from build123d import *

# Parameters (mm, degrees)
SKETCH1_W                = 160
SKETCH1_H                = 60
BOSS_EXTRUDE1_DEPTH      = 5
BOSS_EXTRUDE3_DEPTH      = 14.3
BOSS_EXTRUDE3_DEPTH_BACK = 14.3
SKETCH8_W                = 20
SKETCH8_H                = 23
CUT_EXTRUDE1_REACH       = 134.986
BOSS_EXTRUDE4_DEPTH      = 60
CUT_EXTRUDE2_START       = -71.5
SKETCH11_W               = 45
SKETCH11_H               = 40
CUT_EXTRUDE2_DEPTH       = 71.5
SKETCH12_W               = 24.082620142
SKETCH12_H               = 45
CUT_EXTRUDE3_DEPTH       = 24
SKETCH13_R               = 3.5
SKETCH13_R_2             = 1.7
CUT_EXTRUDE4_DEPTH       = 7.417379858
SKETCH14_R               = 3.5
BOSS_EXTRUDE5_DEPTH      = 60
SKETCH16_W               = 47
SKETCH16_H               = 47.898935067
CUT_EXTRUDE6_DEPTH       = 107.5
CUT_EXTRUDE7_DEPTH       = 28.5
CUT_EXTRUDE7_DEPTH_BACK  = 28.5
SKETCH17_R               = 7


with BuildPart() as part:
    # Sketch1 → Boss-Extrude1 (new body)
    with BuildSketch(Plane(origin=(0, 0, 0), x_dir=(1, 0, 0), z_dir=(0, 1, 0))):
        Rectangle(SKETCH1_W, SKETCH1_H)
    extrude(amount=BOSS_EXTRUDE1_DEPTH)

    # Sketch8 → Boss-Extrude3 (add, two sides: drawn at the far end of the back side and taken through both)
    with BuildSketch(Plane.XY.offset(-BOSS_EXTRUDE3_DEPTH_BACK)):
        with Locations((-37.5, -11.5)):
            Rectangle(SKETCH8_W, SKETCH8_H)
        with BuildLine():
            Line((-45, -18.5), (-30, -18.5))
            ThreePointArc((-30, -18.5), (-28.5, -20), (-30, -21.5))
            Line((-30, -21.5), (-45, -21.5))
            ThreePointArc((-45, -21.5), (-46.5, -20), (-45, -18.5))
        make_face(mode=Mode.SUBTRACT)
        with BuildLine():
            Line((-45, -0.9), (-30, -0.9))
            ThreePointArc((-30, -0.9), (-28.5, -2.4), (-30, -3.9))
            Line((-30, -3.9), (-45, -3.9))
            ThreePointArc((-45, -3.9), (-46.5, -2.4), (-45, -0.9))
        make_face(mode=Mode.SUBTRACT)
    extrude(amount=BOSS_EXTRUDE3_DEPTH + BOSS_EXTRUDE3_DEPTH_BACK)

    # Cut-Extrude1: up to this face of the body (flat: up to its plane)
    cut_extrude1_end = Plane(part.part.faces().sort_by_distance((-27.5, -11.5, 0))[0])
    # Sketch9 → Cut-Extrude1 (cut, up to the picked face)
    with BuildSketch(Plane.ZY.offset(47.5), mode=Mode.PRIVATE) as cut_extrude1_sk1:
        Polygon((-9.3, -23), (9.3, -23), (9.3, 0), (-9.3, 0), (-9.3, -9.4), (-11.3, -9.4), (-11.3, -13.4), (-9.3, -13.4), align=None)
    cut_extrude1_tool1 = split(extrude(cut_extrude1_sk1.sketch, amount=-CUT_EXTRUDE1_REACH, mode=Mode.PRIVATE), bisect_by=cut_extrude1_end, keep=Keep.BOTH, mode=Mode.PRIVATE)
    add(cut_extrude1_tool1.solids().sort_by(Axis((-47.5, -11.498164, -0.189078), (1, 0, 0)))[0], mode=Mode.SUBTRACT)

    # Sketch10 → Boss-Extrude4 (add)
    with BuildSketch(Plane.XY.offset(30)):
        Polygon((-72.5, 69), (-8.5, 5), (-19.106601718, 5), (-70, 55.893398282), (-70, 5), (-72.5, 5), (-80, 5), (-80, 69), align=None)
    extrude(amount=-BOSS_EXTRUDE4_DEPTH)

    # Sketch11 → Cut-Extrude2 (cut)
    with BuildSketch(Plane.ZY.offset(80).offset(CUT_EXTRUDE2_START)):
        with Locations((0, 25)):
            Rectangle(SKETCH11_W, SKETCH11_H)
    extrude(amount=CUT_EXTRUDE2_DEPTH, mode=Mode.SUBTRACT)

    # Sketch12 → Cut-Extrude3 (cut)
    with BuildSketch(Plane(origin=(0, 69, 0), x_dir=(1, 0, 0), z_dir=(0, 1, 0))):
        with Locations((-60.541310071, 0)):
            Rectangle(SKETCH12_W, SKETCH12_H)
    extrude(amount=-CUT_EXTRUDE3_DEPTH, mode=Mode.SUBTRACT)

    # Sketch13 → Cut-Extrude4 (cut)
    with BuildSketch(Plane.ZY.offset(80)):
        with Locations((0, 57)):
            Circle(SKETCH13_R)
        with Locations((-8.5, 57)):
            Circle(SKETCH13_R_2)
        with Locations((8.5, 57)):
            Circle(SKETCH13_R_2)
    extrude(amount=-CUT_EXTRUDE4_DEPTH, mode=Mode.SUBTRACT)

    # Sketch14 → Boss-Extrude5 (add)
    with BuildSketch(Plane.XY.offset(30)):
        with BuildLine():
            Line((80, 0), (66.844135363, -38.995809861))
            ThreePointArc((66.844135363, -38.995809861), (55, -47.500001557), (43.155864637, -38.995809861))
            Line((43.155864637, -38.995809861), (30, 0))
            Line((30, 0), (37.5, 0))
            Line((37.5, 0), (46.28476615, -26.03926689))
            ThreePointArc((46.28476615, -26.03926689), (55, -22.499998443), (63.71523385, -26.03926689))
            Line((63.71523385, -26.03926689), (72.5, 0))
            Line((72.5, 0), (80, 0))
        make_face()
        with Locations((55, -35)):
            Circle(SKETCH14_R, mode=Mode.SUBTRACT)
    extrude(amount=-BOSS_EXTRUDE5_DEPTH)

    # Sketch16 → Cut-Extrude6 (cut)
    with BuildSketch(Plane(origin=(80, 0, 0), x_dir=(0, 0, -1), z_dir=(1, 0, 0))):
        with Locations((0, -23.949467534)):
            Rectangle(SKETCH16_W, SKETCH16_H)
    extrude(amount=-CUT_EXTRUDE6_DEPTH, mode=Mode.SUBTRACT)

    # Sketch17 → Cut-Extrude7 (cut, two sides: drawn at the far end of the back side and taken through both)
    with BuildSketch(Plane.XY.offset(-CUT_EXTRUDE7_DEPTH_BACK)):
        with Locations((55, -35)):
            Circle(SKETCH17_R)
    extrude(amount=CUT_EXTRUDE7_DEPTH + CUT_EXTRUDE7_DEPTH_BACK, mode=Mode.SUBTRACT)


solid = part.part
The listing builds one solid part. Answer for the finished solid, in the listing's coordinates (mm). A direction names the side the tool comes from. Round coordinates to 2 decimals unless told otherwise and drop trailing zeros. Write each loop counter-clockwise with the first axis right and the second up, starting at its lowest first coordinate (ties: lowest second). Pieces come first, ordered by that corner, then holes. Notation, with made-up numbers: M 71,84.25 L 110,84.25 A33 ccw 110,114.25 Z; hole C -23.75,-3.5 d11. An arc over 180 degrees is marked long. Write each question's results on one line, items separated by ' | '. Start each with the question number.
Item 1: For faces 1 (the face through (58, -38, 28.5)), 2 (the face through (-27.5, -12, 12)), 3 (the face through (68.046, -13.202, -26.705)), 4 (the face through (55, -24, -23.5)), 5 (the face through (-76, 45, 0)), determine the directions among +Z, -Z, +X, -X, +Y, -Y from which every point of the face is accessible in a straight line to the end or side of a thin tool.
Item 2: A cutting plane is placed at C-C on x = 53.5. Write down the section's boundary in (y, z).
Item 3: A cutting plane is placed at D-D on x = -58. Write down the section's boundary in (y, z), and give its area (3 significant figures).
Item 4: A cutting plane is placed at B-B on x = -11. Write down the section's boundary in (y, z), and give its area (4 significant figures).
Item 5: Flat-ended cylindrical pins translate along their axes: pin 1 Ø6 at (x, z) = (53.5, -16.5) entering from +Y; pin 2 Ø4 at (y, z) = (19.5, 27) entering from +X; pin 3 Ø5.5 at (x, z) = (-36.5, -11.5) entering from -Y. Find the tip coordinate at first contact, or state that the pin passes through.
Item 6: For a pull along Z with two mould halves and no side action, classify faces 6 (the face through (-38, -12, 9.3)), 7 (the face through (52.42, -32.635, -29.24)), 8 (the face through (-38, -11, -14.3)), 9 (the face through (-72.583, 57, 5)) as pulls with the +Z half, pulls with the -Z half, needs draft (parallel to the pull), parting line crosses it, or undercut.
Item 7: A cutting plane is placed at A-A on y = -35. Write down the section's boundary in (x, z), and give its area (3 significant figures).
Item 8: Straight lines are drawn through the part: L1, parallel to Y at x = 55, z = -24.6; L2, parallel to Y at x = -78.5, z = -8.5; L3, parallel to Y at x = 59, z = 21. For each, find the intervals that lie inside material, in ascending order. Write a range as [from, to].
Check sheet entries:
1) face 1: none | face 2: +Z, -Z, +X, -Y | face 3: +Z, -Z | face 4: +X, -X, -Y | face 5: +X, -X
2) outline: M -47.41,-30 L -38.16,-30 L -38.16,-28.5 L -41.84,-28.5 L -41.84,-23.5 L -47.41,-23.5 Z; M -47.41,23.5 L -41.84,23.5 L -41.84,28.5 L -38.16,28.5 L -38.16,30 L -47.41,30 Z; M -31.84,-30 L -22.59,-30 L -22.59,-23.5 L -28.16,-23.5 L -28.16,-28.5 L -31.84,-28.5 Z; M -31.84,28.5 L -28.16,28.5 L -28.16,23.5 L -22.59,23.5 L -22.59,30 L -31.84,30 Z; M 0,-30 L 5,-30 L 5,30 L 0,30 Z
3) outline: M 0,-30 L 5,-30 L 5,30 L 0,30 Z; M 43.89,-30 L 54.5,-30 L 54.5,-22.5 L 43.89,-22.5 Z; M 43.89,22.5 L 54.5,22.5 L 54.5,30 L 43.89,30 Z | area: 459 mm²
4) outline: M 0,-30 L 7.5,-30 L 7.5,-22.5 L 5,-22.5 L 5,22.5 L 7.5,22.5 L 7.5,30 L 0,30 Z | area: 337.5 mm²
5) pin 1: y = 5 | pin 2: x = -21 | pin 3: y = -23
6) face 6: undercut | face 7: needs draft | face 8: pulls with the -Z half | face 9: undercut
7) outline: M 41.81,-30 L 51.5,-30 L 51.5,-28.5 L 48,-28.5 L 48,-23.5 L 41.81,-23.5 Z; M 41.81,23.5 L 48,23.5 L 48,28.5 L 51.5,28.5 L 51.5,30 L 41.81,30 Z; M 58.5,-30 L 68.19,-30 L 68.19,-23.5 L 62,-23.5 L 62,-28.5 L 58.5,-28.5 Z; M 58.5,28.5 L 62,28.5 L 62,23.5 L 68.19,23.5 L 68.19,30 L 58.5,30 Z | area: 182 mm²
8) L1: [-47.5, -42], [-28, -22.5], [0, 5] | L2: [0, 5], [45, 55.3], [58.7, 69] | L3: [0, 5]
